```python
from build123d import *

# Parameters (mm, degrees)
SKETCH1_W             = 630
SKETCH1_H             = 152.4
BOSS_EXTRUDE1_DEPTH   = 12.7
SKETCH8_W             = 630
SKETCH8_H             = 2.7
CUT_EXTRUDE1_DEPTH    = 351.160034841
BOSS_EXTRUDE2_REACH   = 326.702
M8_CLEARANCE_HOLE1_D  = 9
M20_CLEARANCE_HOLE1_D = 22
M6_TAPPED_HOLE2_D     = 5
M6_TAPPED_HOLE2_DEPTH = 27.99
M6_TAPPED_HOLE2_TIP   = 1.502151548
M6_TAPPED_HOLE5_D     = 5
M6_TAPPED_HOLE5_DEPTH = 27.99
M6_TAPPED_HOLE5_TIP   = 1.502151548
M6_TAPPED_HOLE6_D     = 5
M6_TAPPED_HOLE6_DEPTH = 27.99
M6_TAPPED_HOLE6_TIP   = 1.502151548
M6_TAPPED_HOLE3_D     = 5
M6_TAPPED_HOLE3_DEPTH = 27.99
M6_TAPPED_HOLE3_TIP   = 1.502151548
M6_TAPPED_HOLE7_D     = 5
M6_TAPPED_HOLE7_DEPTH = 27.99
M6_TAPPED_HOLE7_TIP   = 1.502151548
M6_TAPPED_HOLE8_D     = 5
M6_TAPPED_HOLE8_DEPTH = 27.99
M6_TAPPED_HOLE8_TIP   = 1.502151548
FILLET1_R             = 0.79375


with BuildPart() as part:
    # Sketch1 → Boss-Extrude1 (new, symmetric)
    with BuildSketch(Plane(origin=(0, 0, 0), x_dir=(1, 0, 0), z_dir=(0, 1, 0))):
        Rectangle(SKETCH1_W, SKETCH1_H)
    extrude(amount=BOSS_EXTRUDE1_DEPTH, both=True)

    # Sketch8 → Cut-Extrude1 (cut, through all)
    with BuildSketch(Plane(origin=(0, 0, 76.2), x_dir=(-1, 0, 0), z_dir=(0, 0, -1))):
        Polygon((-83.2, -10), (-83.2, -4), (-68.9125, -4), (-68.9125, -10), (116.8, -10), (116.8, -4), (131.0875, -4), (131.0875, -10), (315, -10), (315, -12.7), (-315, -12.7), (-315, -10), (-283.2, -10), (-283.2, -4), (-268.9125, -4), (-268.9125, -10), align=None)
        with Locations((0, 11.35)):
            Rectangle(SKETCH8_W, SKETCH8_H)
    extrude(amount=CUT_EXTRUDE1_DEPTH, mode=Mode.SUBTRACT)

    # Sketch23 → Boss-Extrude2 (add, up to next)
    with BuildSketch(Plane.XZ.offset(10), mode=Mode.PRIVATE) as boss_extrude2_sk1:
        with BuildLine():
            Line((-116.8, 6.35), (-116.8, -76.2))
            Line((-116.8, -76.2), (-131.0875, -76.2))
            Line((-131.0875, -76.2), (-131.0875, 6.35))
            ThreePointArc((-131.0875, 6.35), (-123.94375, -0.79375), (-116.8, 6.35))
        make_face()
    boss_extrude2_tool1 = extrude(boss_extrude2_sk1.sketch, amount=-BOSS_EXTRUDE2_REACH, mode=Mode.PRIVATE) - part.part
    # Sketch23 → Boss-Extrude2 (add, up to next)
    with BuildSketch(Plane.XZ.offset(10), mode=Mode.PRIVATE) as boss_extrude2_sk2:
        with BuildLine():
            Line((68.9125, 6.35), (68.9125, -76.2))
            Line((68.9125, -76.2), (83.2, -76.2))
            Line((83.2, -76.2), (83.2, 6.35))
            ThreePointArc((83.2, 6.35), (76.05625, -0.79375), (68.9125, 6.35))
        make_face()
    boss_extrude2_tool2 = extrude(boss_extrude2_sk2.sketch, amount=-BOSS_EXTRUDE2_REACH, mode=Mode.PRIVATE) - part.part
    # Sketch23 → Boss-Extrude2 (add, up to next)
    with BuildSketch(Plane.XZ.offset(10), mode=Mode.PRIVATE) as boss_extrude2_sk3:
        with BuildLine():
            Line((268.9125, 6.35), (268.9125, -76.2))
            Line((268.9125, -76.2), (283.2, -76.2))
            Line((283.2, -76.2), (283.2, 6.35))
            ThreePointArc((283.2, 6.35), (276.05625, -0.79375), (268.9125, 6.35))
        make_face()
    boss_extrude2_tool3 = extrude(boss_extrude2_sk3.sketch, amount=-BOSS_EXTRUDE2_REACH, mode=Mode.PRIVATE) - part.part
    add(boss_extrude2_tool1.solids().sort_by_distance((-123.94375, -10, -37.713823))[0])
    add(boss_extrude2_tool2.solids().sort_by_distance((76.05625, -10, -37.713823))[0])
    add(boss_extrude2_tool3.solids().sort_by_distance((276.05625, -10, -37.713823))[0])

    # M8 Clearance Hole1 (through all)
    with Locations(Plane(origin=(-252.085824098, -10, 54.789326217), x_dir=(-1, 0, 0), z_dir=(0, -1, 0))):
        with Locations((47.914175902, 109.589326217), (-52.085824098, 109.589326217), (-152.085824098, 59.589326217), (-252.085824098, 109.589326217), (-352.085824098, 59.589326217), (-452.085824098, 109.589326217), (-552.085824098, 109.589326217)):
            Hole(M8_CLEARANCE_HOLE1_D / 2)

    # M20 Clearance Hole1 (through all)
    with Locations(Plane(origin=(-106.699185936, -10, 17.134873145), x_dir=(-1, 0, 0), z_dir=(0, -1, 0))):
        with Locations((193.300814064, 21.934873145), (-406.699185936, 21.934873145), (-206.699185936, 71.934873145), (-6.699185936, 71.934873145)):
            Hole(M20_CLEARANCE_HOLE1_D / 2)

    # M6 Tapped Hole2
    with Locations(Plane(origin=(-22.829775721, -10, 14.438586314), x_dir=(-1, 0, 0), z_dir=(0, -1, 0))):
        with Locations((-155.829775721, -4.761413686), (-208.829775721, 19.238586314), (-155.829775721, 19.238586314), (-208.829775721, -4.761413686), (-229.829775721, -49.761413686), (-286.829775721, -4.761413686), (-229.829775721, -4.761413686), (-286.829775721, -49.761413686)):
            Hole(M6_TAPPED_HOLE2_D / 2, depth=M6_TAPPED_HOLE2_DEPTH)
            with Locations((0, 0, -(M6_TAPPED_HOLE2_DEPTH + M6_TAPPED_HOLE2_TIP / 2))):  # 118° drill point
                Cone(0, M6_TAPPED_HOLE2_D / 2, M6_TAPPED_HOLE2_TIP, mode=Mode.SUBTRACT)

    # M6 Tapped Hole5
    with Locations(Plane(origin=(0, -10, 0), x_dir=(-1, 0, 0), z_dir=(0, -1, 0))):
        with Locations((14, 4.8), (67, -19.2), (14, -19.2), (67, 4.8), (-64, -19.2), (-7, -64.2), (-64, -64.2), (-7, -19.2)):
            Hole(M6_TAPPED_HOLE5_D / 2, depth=M6_TAPPED_HOLE5_DEPTH)
            with Locations((0, 0, -(M6_TAPPED_HOLE5_DEPTH + M6_TAPPED_HOLE5_TIP / 2))):  # 118° drill point
                Cone(0, M6_TAPPED_HOLE5_D / 2, M6_TAPPED_HOLE5_TIP, mode=Mode.SUBTRACT)

    # M6 Tapped Hole6
    with Locations(Plane(origin=(0, -10, 0), x_dir=(-1, 0, 0), z_dir=(0, -1, 0))):
        with Locations((136, -19.2), (193, -64.2), (136, -64.2), (193, -19.2), (214, 4.8), (267, -19.2), (214, -19.2), (267, 4.8)):
            Hole(M6_TAPPED_HOLE6_D / 2, depth=M6_TAPPED_HOLE6_DEPTH)
            with Locations((0, 0, -(M6_TAPPED_HOLE6_DEPTH + M6_TAPPED_HOLE6_TIP / 2))):  # 118° drill point
                Cone(0, M6_TAPPED_HOLE6_D / 2, M6_TAPPED_HOLE6_TIP, mode=Mode.SUBTRACT)

    # M6 Tapped Hole3
    with Locations(Plane(origin=(0, -4, 0), x_dir=(-1, 0, 0), z_dir=(0, -1, 0))):
        with Locations((-276.85, -19.2), (-276.85, -64.2)):
            Hole(M6_TAPPED_HOLE3_D / 2, depth=M6_TAPPED_HOLE3_DEPTH)
            with Locations((0, 0, -(M6_TAPPED_HOLE3_DEPTH + M6_TAPPED_HOLE3_TIP / 2))):  # 118° drill point
                Cone(0, M6_TAPPED_HOLE3_D / 2, M6_TAPPED_HOLE3_TIP, mode=Mode.SUBTRACT)

    # M6 Tapped Hole7
    with Locations(Plane(origin=(0, -4, 0), x_dir=(-1, 0, 0), z_dir=(0, -1, 0))):
        with Locations((-76.85, -19.2), (-76.85, -64.2)):
            Hole(M6_TAPPED_HOLE7_D / 2, depth=M6_TAPPED_HOLE7_DEPTH)
            with Locations((0, 0, -(M6_TAPPED_HOLE7_DEPTH + M6_TAPPED_HOLE7_TIP / 2))):  # 118° drill point
                Cone(0, M6_TAPPED_HOLE7_D / 2, M6_TAPPED_HOLE7_TIP, mode=Mode.SUBTRACT)

    # M6 Tapped Hole8
    with Locations(Plane(origin=(0, -4, 0), x_dir=(-1, 0, 0), z_dir=(0, -1, 0))):
        with Locations((123.15, -19.2), (123.15, -64.2)):
            Hole(M6_TAPPED_HOLE8_D / 2, depth=M6_TAPPED_HOLE8_DEPTH)
            with Locations((0, 0, -(M6_TAPPED_HOLE8_DEPTH + M6_TAPPED_HOLE8_TIP / 2))):  # 118° drill point
                Cone(0, M6_TAPPED_HOLE8_D / 2, M6_TAPPED_HOLE8_TIP, mode=Mode.SUBTRACT)

    # Fillet1
    fillet1_edges = [part.edges().sort_by_distance(p)[0] for p in [
        (283.2, -4, 41.275),
        (268.9125, -4, 41.275),
        (276.05625, -4, -0.79375),
        (-116.8, -4, 41.275),
        (-131.0875, -4, 41.275),
        (-123.94375, -4, -0.79375),
        (83.2, -4, 41.275),
        (68.9125, -4, 41.275),
        (76.05625, -4, -0.79375),
    ]]
    fillet(fillet1_edges, radius=FILLET1_R)


solid = part.part
```
CAD build for the part. Positions are in the model's coordinates, mm. A direction names the side the tool comes from. Round coordinates to 2 decimals unless told otherwise and drop trailing zeros. Return JSON: item names as keys, results as strings. Group by question number.
Item 1: Flat gauge pins, fed straight in: pin 1 Ø2 at (x, y) = (78, -5.5) entering from +Z; pin 2 Ø8 at (x, z) = (186, -4.8) entering from +Y; pin 3 Ø6.5 at (x, z) = (-123.15, 19.2) entering from -Y. Where does each tip first touch, or does it go through?
Item 2: Probe probe 1 along Z at (x, y) = (-214, 2); probe 2 along X at (y, z) = (-7.25, 33); probe 3 along Z at (x, y) = (264, 2.5). List the from-to ranges inside material, lowest first.
Item 3: Band-saw the part on A-A on y = 6. State how many separate pieces and enclosed holes the cut face has, plus the area to 3 significant figures.
Item 4: 3-axis set-ups, long thin cutter, end or side, ignore diameter. For faces 1 (the face through (-311, 0, -5)), 2 (the face through (76, -4, 39)): which of +Z, -Z, +X, -X, +Y, -Y reach the whole face in a straight line?
Item 5: Mould opens along Z. For faces 3 (the face through (-4, 0, -76.2)), 4 (the face through (89, 0, -55)), 5 (the face through (276, -4, 39)) say: +Z half, -Z half, draft (parallel to the pull), parting line (faces both ways), or undercut.
Resolved:
{
 "1": {"pin 1": "stops at z = -0.16", "pin 2": "stops at y = 10", "pin 3": "stops at y = -4"},
 "2": {"probe 1": "z = -76.2 to -7.3, -2.3 to 16.7, 21.7 to 76.2", "probe 2": "x = -315 to -131.09, -116.8 to 68.91, 83.2 to 268.91, 283.2 to 315", "probe 3": "z = -76.2 to 16.7, 21.7 to 61.7, 66.7 to 76.2"},
 "3": {"separate pieces": "1", "enclosed holes": "41", "area": "93,500 mm²"},
 "4": {"face 1": "+Y, -Y", "face 2": "+Z, -Y"},
 "5": {"face 3": "-Z half", "face 4": "undercut", "face 5": "draft"}
}
